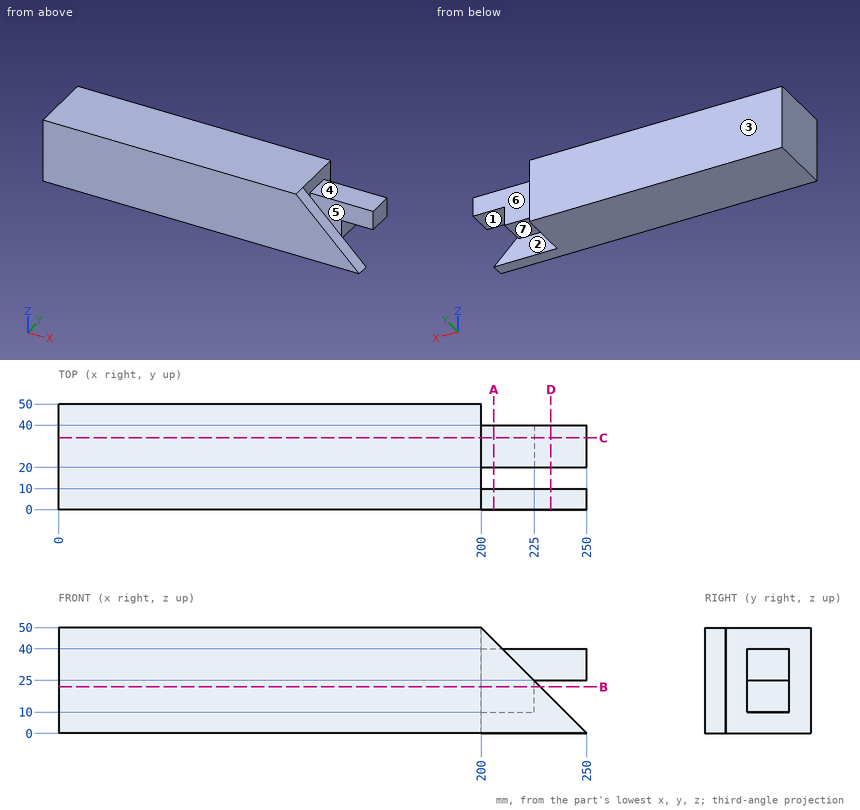
Here's the drawing with two shaded views (mm, measured from the low corner). I have some questions. A direction names the side the tool comes from. Give positions to 0.01 mm unless a question says otherwise; leave off trailing zeros. Order: outer loops, then holes, each group sorted by start corner. A loop starts at its lowest first (then second) coordinate and runs counter-clockwise, first axis right, second up. Notation, with made-up numbers: M 26.25,-36 L 44.25,-36 A14 ccw 44.25,-23 Z; hole C -33,-1 d3. An arc over 180 degrees is marked long. Answer as a JSON object with one key per item and string values. Group by question number.
1) Please list where these lines run through material, in increasing order: L1, parallel to Y at x = 228.5, z = 8.5; L2, parallel to X at y = 45, z = 29.5; L3, parallel to X at y = 23.5, z = 20.5. Write a range as [from, to].
2) Suppose I cut it at D-D, the plane x = 233. Write out the boundary of the cut face in (y, z).
3) We'd pull the mould along Y, two halves only. Please class the marked faces 1, 2 and 3: pulls with the +Y half, pulls with the -Y half, needs draft (parallel to the pull), parting line crosses it, or undercut.
4) Suppose I cut it at A-A, the plane x = 206. Write out the boundary of the cut face in (y, z).
5) Suppose I cut it at B-B, the plane z = 22. Write out the boundary of the cut face in (x, y), plus the area to 3 significant figures.
6) Suppose I cut it at C-C, the plane y = 34. Write out the boundary of the cut face in (x, z), plus the area to 3 significant figures.
7) I'm going to push flat-ended pins straight in: pin 1 Ø1.5 at (y, z) = (14.5, 9) entering from +X; pin 2 Ø25 at (x, z) = (221, 30) entering from +Y; pin 3 Ø6 at (y, z) = (28, 14) entering from +X. Where does each tip first touch, or does it pass through?
8) On a 3-axis mill with a long thin cutter (end or side, diameter ignored), from which of +Z, -Z, +X, -X, +Y, -Y can I reach the whole of each face in a straight line? I mean the marked faces 4, 5, 6 and 7. Say none if no direction works.
Results found:
{
 "1": {"L1": "[0, 10]", "L2": "[0, 200]", "L3": "[0, 225]"},
 "2": {"outline": "M 0,0 L 10,0 L 10,17 L 0,17 Z; M 20,25 L 40,25 L 40,40 L 20,40 Z"},
 "3": {"face 1": "needs draft", "face 2": "undercut", "face 3": "pulls with the +Y half"},
 "4": {"outline": "M 0,0 L 10,0 L 10,44 L 0,44 Z; M 20,10 L 40,10 L 40,40 L 20,40 Z"},
 "5": {"outline": "M 0,0 L 228,0 L 228,10 L 200,10 L 200,20 L 225,20 L 225,40 L 200,40 L 200,50 L 0,50 Z", "area": "10,800 mm²"},
 "6": {"outline": "M 0,0 L 200,0 L 200,10 L 225,10 L 225,25 L 250,25 L 250,40 L 200,40 L 200,50 L 0,50 Z", "area": "11,100 mm²"},
 "7": {"pin 1": "x = 200", "pin 2": "y = 40", "pin 3": "x = 225"},
 "8": {"face 4": "+Z, +X, +Y", "face 5": "+Z, -Z, +X", "face 6": "+Z, -Z, +X, +Y", "face 7": "-Z, +X, +Y"}
}
